from build123d import *

# Parameters (mm, degrees)
SKETCH1_R           = 19
SKETCH1_R_2         = 12.85
SKETCH1_R_3         = 2
BOSS_EXTRUDE1_DEPTH = 3


with BuildPart() as part:
    # Sketch1 → Boss-Extrude1 (new body)
    with BuildSketch(Plane(origin=(0, 0, 0), x_dir=(1, 0, 0), z_dir=(0, 1, 0))):
        Circle(SKETCH1_R)
        Circle(SKETCH1_R_2, mode=Mode.SUBTRACT)
        with Locations((-9.586926691, 12.809794558)):
            Circle(SKETCH1_R_3, mode=Mode.SUBTRACT)
        with Locations((12.809794558, 9.586926691)):
            Circle(SKETCH1_R_3, mode=Mode.SUBTRACT)
        with Locations((9.586926691, -12.809794558)):
            Circle(SKETCH1_R_3, mode=Mode.SUBTRACT)
        with BuildLine():
            Line((-11.812857964, -12.587946089), (-15.407955473, -7.784273129))
            ThreePointArc((-15.407955473, -7.784273129), (-15.206526231, -6.384478051), (-13.806731153, -6.585907293))
            Line((-13.806731153, -6.585907293), (-10.211633644, -11.389580252))
            ThreePointArc((-10.211633644, -11.389580252), (-10.413062886, -12.78937533), (-11.812857964, -12.587946089))
        make_face(mode=Mode.SUBTRACT)
    extrude(amount=BOSS_EXTRUDE1_DEPTH)


solid = part.part
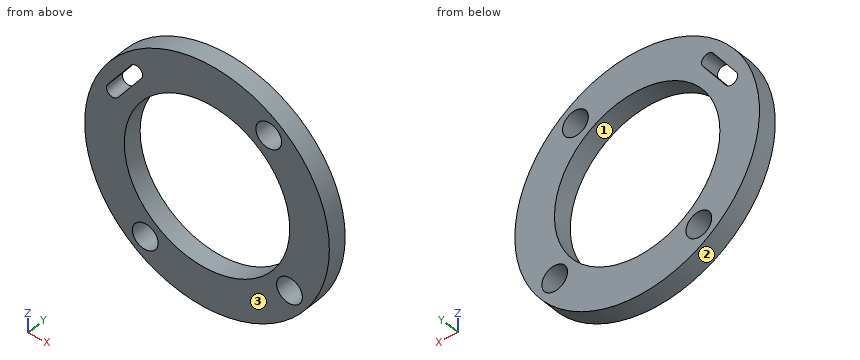
Here's how the part is built. I have some questions about the finished solid (model axes, mm). Face numbers are marked on the shaded views. Give positions to 0.01 mm unless a question says otherwise; leave off trailing zeros. Loops run counter-clockwise (first coordinate to the right, second up) from the corner with the lowest first, then second, coordinate; pieces in that order, holes last. Notation, with made-up numbers: (12.5, -30) -> (16.5, -30) arc R23 cw to (16.5, -2) -> close; hole circle Ø10 at (-3.5, -26.5). An arc over 180 degrees is marked (long way). Answer as a JSON object with one key per item and string values. Group by question number.
Item 1: Imagine slicing it at D-D on z = -8.5. Write out the boundary of the cut face in (x, y).
Item 2: Imagine slicing it at A-A on x = 0. Write out the boundary of the cut face in (y, z).
Item 3: Imagine slicing it at C-C on y = 2.25. Write out the boundary of the cut face in (x, z).
Item 4: Thinking about a two-plate mould opening in Z: for the marked faces 1, 2 and 3, which applies, pulls with the +Z half, pulls with the -Z half, needs draft (parallel to the pull), parting line crosses it, or undercut?
Item 5: Imagine slicing it at B-B on z = 0. Write out the boundary of the cut face in (x, y), then the cut area to 3 significant figures.
Item 6: Will these pins go through, and if not, where does the flat tip stop? pin 1 (4.5 mm diameter, centred on x = 9.59, z = 12.81, fed in from -Y); pin 2 (2.5 mm diameter, centred on x = 12.81, z = -9.59, fed in from -Y); pin 3 (1 mm diameter, centred on y = 0.5, z = -9.5, fed in from -X); pin 4 (1 mm diameter, centred on y = 0.5, z = 3, fed in from -X).
Item 7: I need wall thicknesses on L1, parallel to Z at x = 0, y = 2.25; L2, parallel to Z at x = 8.5, y = 1.5; L3, parallel to Z at x = 8, y = 1.9. Which ranges of each line are inside material? Lowest first, please.
Answer list:
{
 "1": {"outline": "(-16.99, 0) -> (-9.64, 0) -> (-9.64, 3) -> (-16.99, 3) -> close; (9.64, 0) -> (11.13, 0) -> (11.13, 3) -> (9.64, 3) -> close; (14.49, 0) -> (16.99, 0) -> (16.99, 3) -> (14.49, 3) -> close"},
 "2": {"outline": "(0, -19) -> (3, -19) -> (3, -12.85) -> (0, -12.85) -> close; (0, 12.85) -> (3, 12.85) -> (3, 19) -> (0, 19) -> close"},
 "3": {"outline": "circle Ø38 at (0, 0); hole (-15.41, 7.78) arc R1 ccw to (-13.81, 6.59) -> (-10.21, 11.39) arc R1 ccw to (-11.81, 12.59) -> close; hole circle Ø25.7 at (0, 0); hole circle Ø4 at (-9.59, -12.81); hole circle Ø4 at (9.59, 12.81); hole circle Ø4 at (12.81, -9.59)"},
 "4": {"face 1": "undercut", "face 2": "parting line crosses it", "face 3": "needs draft"},
 "5": {"outline": "(-19, 0) -> (-12.85, 0) -> (-12.85, 3) -> (-19, 3) -> close; (12.85, 0) -> (19, 0) -> (19, 3) -> (12.85, 3) -> close", "area": "36.9 mm2"},
 "6": {"pin 1": "stops at y = 0", "pin 2": "passes through", "pin 3": "stops at x = -16.73", "pin 4": "stops at x = -18.83"},
 "7": {"L1": "z = -19 to -12.85, 12.85 to 19", "L2": "z = -16.99 to -9.64, 9.64 to 11.13, 14.49 to 16.99", "L3": "z = -17.23 to -10.06, 10.06 to 11.59, 14.03 to 17.23"}
}
